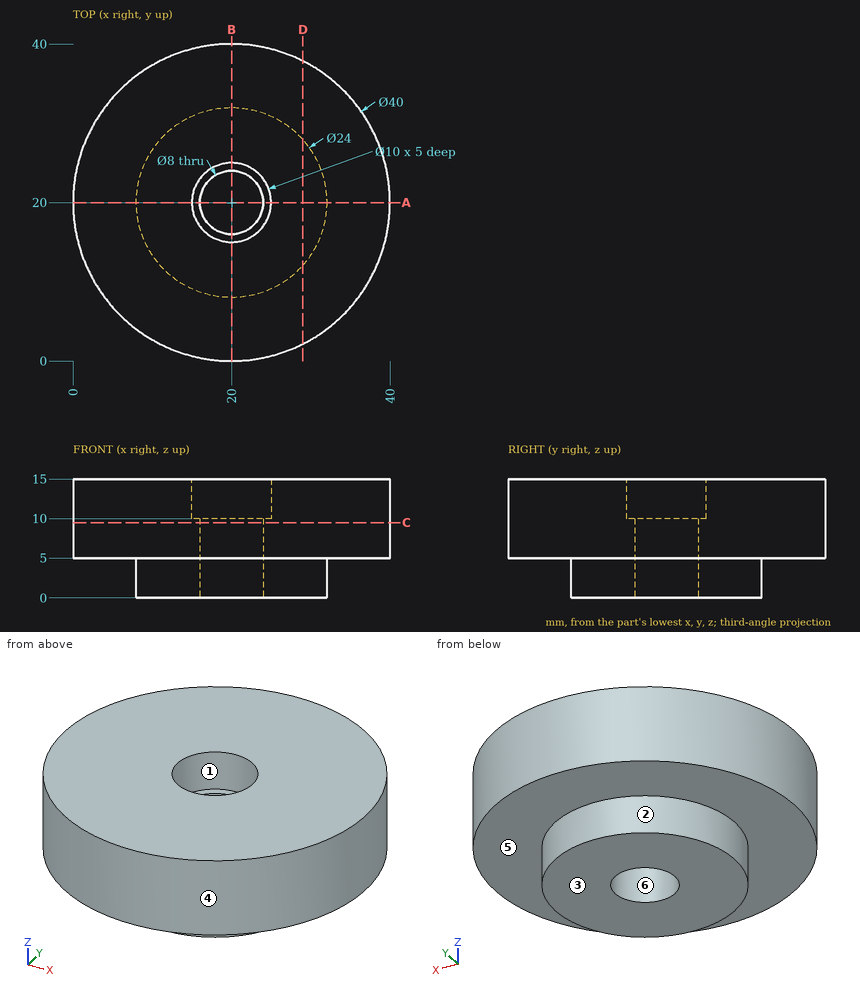
For this review, use the dimensioned drawing (mm, ordinates from the lowest corner) and the shaded views. A direction names the side the tool comes from. Round coordinates to 2 decimals unless told otherwise and drop trailing zeros. Order: outer loops, then holes, each group sorted by start corner. A loop starts at its lowest first (then second) coordinate and runs counter-clockwise, first axis right, second up. Notation, with made-up numbers: M -34,2.5 L 24,2.5 A20 ccw 24,18.5 Z; hole C -36.5,-1 d10. An arc over 180 degrees is marked long. Use a Markdown table: item, result.
1) Consider section D-D (x = 29). Write out the cut boundary in (y, z).
Report:
| item | result |
|---|---|
| outline | M 2.14,5 L 12.06,5 L 12.06,0 L 27.94,0 L 27.94,5 L 37.86,5 L 37.86,15 L 2.14,15 Z |
2) Wall thickness on line 1 along Y through (x, z) = (20, 13.9); line 2 along Y through (x, z) = (20, 7); line 3 along X through (y, z) = (20, 2.75): over which ranges is each line inside the solid? List them lowest first. Write a range as [from, to].
Report:
| item | result |
|---|---|
| line 1 | [0, 15], [25, 40] |
| line 2 | [0, 16], [24, 40] |
| line 3 | [8, 16], [24, 32] |
3) Consider section A-A (y = 20). Write out the cut boundary in (x, z), then the cut area to 3 significant figures.
Report:
| item | result |
|---|---|
| outline | M 0,5 L 8,5 L 8,0 L 16,0 L 16,10 L 15,10 L 15,15 L 0,15 Z; M 24,0 L 32,0 L 32,5 L 40,5 L 40,15 L 25,15 L 25,10 L 24,10 Z |
| area | 390 mm^2 |
4) Insertion check: pin 1 (2 mm diameter, centred on y = 15.5, z = 3.5, fed in from -X); pin 2 (4 mm diameter, centred on x = 6, z = 13, fed in from +Y); pin 3 (4 mm diameter, centred on x = 28.5, z = 12.5, fed in from +Y). Each pin has a flat end and moves straight along its axis. Give the tip position at first contact, or say it passes through.
Report:
| item | result |
|---|---|
| pin 1 | x = 8.52 |
| pin 2 | y = 36 |
| pin 3 | y = 38.91 |
5) Draft analysis for pull direction X (two halves, no side actions). For the marked faces 4, 5 and 6, state which applies: released by +X, released by -X, zero draft, split by the parting line, or undercut.
Report:
| item | result |
|---|---|
| face 4 | split by the parting line |
| face 5 | zero draft |
| face 6 | undercut |
6) Consider section C-C (z = 9.5). Write out the cut boundary in (x, y).
Report:
| item | result |
|---|---|
| outline | C 20,20 d40; hole C 20,20 d8 |
7) Tool access review of the marked faces 1, 2 and 3: name each direction out of +Z, -Z, +X, -X, +Y, -Y from which nothing blocks a thin tool from reaching the whole face with its end or side.
Report:
| item | result |
|---|---|
| face 1 | +Z |
| face 2 | -Z |
| face 3 | -Z, +X, -X, +Y, -Y |
